Input: part model. Units: mm. Frame: model coordinates. Coordinates: 2 decimals unless noted, no trailing zeros. Write each loop counter-clockwise with the first axis right and the second up, starting at its lowest first coordinate (ties: lowest second). Pieces come first, ordered by that corner, then holes. Notation, with made-up numbers: M 46.25,39 L 60.25,39 A22 cw 60.25,57 Z; hole C 31.5,56.5 d7. An arc over 180 degrees is marked long. Use one line per item in the form item = value.
from build123d import *

# Parameters (mm, degrees)
F0_R     = 2.5
F1_DEPTH = 1.25
F2_R     = 2.49999
F3_SIZE  = 1.5


# Not quite as in the source:
# - a fillet or chamfer is up to 0.001 mm smaller than in the source, because OpenCascade refuses the exact size


with BuildPart() as f1:
    # F0 (on Top) → F1 (new body, symmetric)
    with BuildSketch(Plane.XY):
        Polygon((41.4535664022, 86.8200212717), (-41.4534695446, 86.8200212717), (-41.4534695446, -23.9119753242), (21.4531961828, -86.8199840188), (41.4535664022, -86.8199840188), align=None)
        with Locations((-36.4534695446, -8.1799787283)):
            Circle(F0_R, mode=Mode.SUBTRACT)
        with Locations((36.4535664022, -71.8299787283)):
            Circle(F0_R, mode=Mode.SUBTRACT)
        with Locations((36.4535664022, -1.2799787283)):
            Circle(F0_R, mode=Mode.SUBTRACT)
        with BuildLine():
            Line((-20.7270524408, -3.1985588427), (-20.7270524408, 69.3289190531))
            ThreePointArc((-20.7270524408, 69.3289190531), (-17.1909272701, 67.8581418384), (-15.7270524408, 64.3191536607))
            Line((-15.7270524408, 64.3191536607), (-15.7270524408, -8.1787062808))
            ThreePointArc((-15.7270524408, -8.1787062808), (-19.2613774966, -6.7270807891), (-20.7270524408, -3.1985588427))
        make_face(mode=Mode.SUBTRACT)
        with BuildLine():
            Line((-2.5020524408, -3.1985588427), (-2.5020524408, 69.3289190531))
            ThreePointArc((-2.5020524408, 69.3289190531), (1.0340727299, 67.8581418384), (2.4979475592, 64.3191536607))
            Line((2.4979475592, 64.3191536607), (2.4979475592, -8.1787062808))
            ThreePointArc((2.4979475592, -8.1787062808), (-1.0363774966, -6.7270807891), (-2.5020524408, -3.1985588427))
        make_face(mode=Mode.SUBTRACT)
        with Locations((-36.4534695446, 69.3200212717)):
            Circle(F0_R, mode=Mode.SUBTRACT)
        with BuildLine():
            Line((15.7229475592, -3.1985588427), (15.7229475592, 69.3289190531))
            ThreePointArc((15.7229475592, 69.3289190531), (19.2590727299, 67.8581418384), (20.7229475592, 64.3191536607))
            Line((20.7229475592, 64.3191536607), (20.7229475592, -8.1787062808))
            ThreePointArc((20.7229475592, -8.1787062808), (17.1886225034, -6.7270807891), (15.7229475592, -3.1985588427))
        make_face(mode=Mode.SUBTRACT)
        with Locations((36.4535664022, 69.3200212717)):
            Circle(F0_R, mode=Mode.SUBTRACT)
    extrude(amount=F1_DEPTH, both=True)

    # F2 (radius 2.5 in the source; OpenCascade refuses exactly that, so slightly less here)
    f2_edges = [f1.edges().sort_by_distance(p)[0] for p in [
        (4.8e-05, 86.820021, -1.25),
        (-2.502052, 33.06518, -1.25),
        (2.497948, 28.070224, -1.25),
        (-20.727052, 33.06518, -1.25),
        (-15.727052, 28.070224, -1.25),
        (15.722948, 33.06518, -1.25),
        (20.722948, 28.070224, -1.25),
    ]]
    fillet(f2_edges, radius=F2_R)

    # F3
    f3_edges = [f1.edges().sort_by_distance(p)[0] for p in [
        (-38.95347, 69.320021, -1.25),
        (33.953566, 69.320021, -1.25),
        (33.953566, -1.279979, -1.25),
        (-38.95347, -8.179979, -1.25),
        (33.953566, -71.829979, -1.25),
    ]]
    chamfer(f3_edges, length=F3_SIZE)


solid = f1.part
(1) Line query: probe 1 along X at (y, z) = (11.5, -0.2); probe 2 along X at (y, z) = (38, 0.8); probe 3 along Y at (x, z) = (19, -0.75). Output: solid intervals per line, ascending.
Computed:
probe_1 = -41.45 to -21.19, -15.26 to -2.97, 2.96 to 15.26, 21.19 to 41.45
probe_2 = -41.45 to -20.77, -15.69 to -2.54, 2.54 to 15.68, 20.76 to 41.45
probe_3 = -84.37 to -8.93, 69.35 to 85.82
(2) Section query C-C on y = -59. Return the cut outline in (x, z), plus the area to 3 significant figures.
Computed:
outline = M -6.37,-1.25 L 41.45,-1.25 L 41.45,1.25 L -6.37,1.25 Z
area = 120 mm^2
(3) Pull-direction query (Y, two-part tool) for faces 1 (the cylindrical face through (38.76, -2.24, 0.74)), 2 (the flat face through (-10.44, -54.926, 0.018)), 3 (the flat face through (9, 0, -1.25)); classes: pulls with the +Y half, pulls with the -Y half, needs draft (parallel to the pull), parting line crosses it, or undercut.
Computed:
face_1 = undercut
face_2 = pulls with the -Y half
face_3 = needs draft
(4) First-contact query: pin 1 Ø1 at (x, z) = (-0.5, -0.5) entering from +Y; pin 2 Ø6.5 at (x, y) = (-36.45, 69.32) entering from -Z. Flat tips, straight axial feed; report the tip coordinate or a pass-through.
Computed:
pin_1 = 86.49
pin_2 = -0.5
(5) Section query A-A on y = 26. State how many separate pieces and enclosed holes the cut face has, plus the area to 3 significant figures.
Computed:
separate_pieces = 4
enclosed_holes = 0
area = 162 mm^2
